The listing builds one solid part. Answer for the finished solid, in the listing's coordinates (mm). Round coordinates to 2 decimals unless told otherwise and drop trailing zeros. Write each loop counter-clockwise with the first axis right and the second up, starting at its lowest first coordinate (ties: lowest second). Pieces come first, ordered by that corner, then holes. Notation, with made-up numbers: M 39.25,-18 L 50.25,-18 A12 cw 50.25,-4 Z; hole C 16.5,-13 d1. An arc over 180 degrees is marked long. Put each result on its own line as item: value. Start each with the question number.
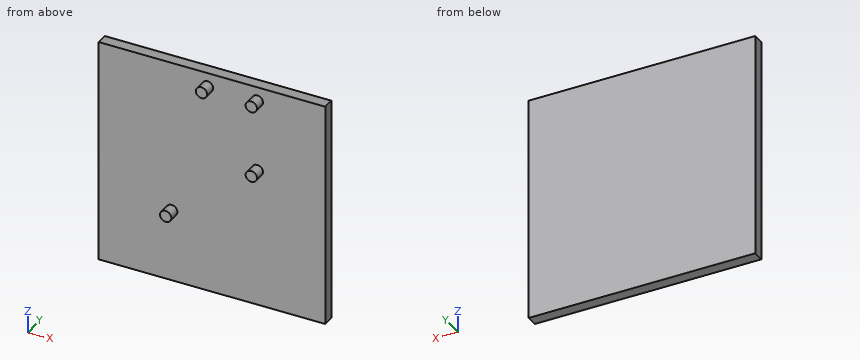
```python
from build123d import *

# Parameters (mm, degrees)
F0_W     = 500
F0_H     = 500
F1_DEPTH = 25
F2_R     = 12.5
F3_DEPTH = 25


with BuildPart() as f1:
    # F0 (on Front) → F1 (new body)
    with BuildSketch(Plane.XZ):
        Rectangle(F0_W, F0_H)
    extrude(amount=F1_DEPTH)

    # F2 (on face) → F3 (join)
    with BuildSketch(Plane.XZ.offset(25)):
        with Locations((-9.894066, 218.870133)):
            Circle(F2_R)
        with Locations((100.105934, 218.870133)):
            Circle(F2_R)
        with Locations((100.105934, 58.870133)):
            Circle(F2_R)
        with Locations((-88.803142, -89.161488)):
            Circle(F2_R)
    extrude(amount=F3_DEPTH)


solid = f1.part
```
Item 1: A flat-ended cylindrical pin translates along its axis: pin 1 (4 mm diameter, centred on x = 8.5, z = 13, fed in from -Y). Find the tip coordinate at first contact, or state that the pin passes through.
Item 2: Section B-B (x = -187) is taken. Give the vertices of the cut face in (y, z), and give its area (3 significant figures).
Item 3: Section C-C (z = 174.5) is taken. Give the vertices of the cut face in (x, y), and give its area (3 significant figures).
Item 4: Consider line 1 along X through (y, z) = (-38, 219); line 2 along Y through (x, z) = (158.5, -192). Determine where each line is inside the solid, lowest interval first. Write a range as [from, to].
Item 5: Section A-A (y = -33) is taken. Give the vertices of the cut face in (x, z).
Output values:
1. pin 1: stops at y = -25
2. outline: M -25,-250 L 0,-250 L 0,250 L -25,250 Z
2. area: 12,500 mm^2
3. outline: M -250,-25 L 250,-25 L 250,0 L -250,0 Z
3. area: 12,500 mm^2
4. line 1: x = [-22.39, 2.61], [87.61, 112.61]
4. line 2: y = [-25, 0]
5. outline: C -88.8,-89.16 d25; C -9.89,218.87 d25; C 100.11,58.87 d25; C 100.11,218.87 d25
